from build123d import *

# Parameters (mm, degrees)
SKETCH1_W                                  = 120
SKETCH1_H                                  = 60
BOSS_EXTRUDE1_DEPTH                        = 10
CUT_EXTRUDE1_DEPTH                         = 71
CUT_EXTRUDE1_DEPTH_BACK                    = 71
SKETCH2_W                                  = 100
SKETCH2_H                                  = 10
FILLET1_R                                  = 5
SKETCH4_R                                  = 1.7
CUT_EXTRUDE3_DEPTH                         = 115.455231423
CUT_EXTRUDE4_DEPTH                         = 3
MIRROR1_AT_THE_SECOND_PLANE_COPY_1_SKETC_R = 1.7
MIRROR1_AT_THE_SECOND_PLANE_COPY_1_DEPTH   = 115.455231423
MIRROR1_AT_THE_SECOND_PLANE_COPY_2_DEPTH   = 3
MIRROR2_COPY_1_SKETCH_R                    = 1.7
MIRROR2_COPY_1_DEPTH                       = 115.455231423
MIRROR2_COPY_2_DEPTH                       = 3
MIRROR2_COPY_3_SKETCH_R                    = 1.7
MIRROR2_COPY_3_DEPTH                       = 115.455231423
MIRROR2_COPY_4_DEPTH                       = 3
MIRROR2_COPY_5_SKETCH_R                    = 1.7
MIRROR2_COPY_5_DEPTH                       = 115.455231423
MIRROR2_COPY_6_DEPTH                       = 3
MIRROR2_COPY_7_SKETCH_R                    = 1.7
MIRROR2_COPY_7_DEPTH                       = 115.455231423
SKETCH6_R                                  = 10
CUT_EXTRUDE5_DEPTH                         = 71


with BuildPart() as part:
    # Sketch1 → Boss-Extrude1 (new, symmetric)
    with BuildSketch(Plane.XY):
        Rectangle(SKETCH1_W, SKETCH1_H)
    extrude(amount=BOSS_EXTRUDE1_DEPTH, both=True)

    # Sketch2 → Cut-Extrude1 (cut, two sides: drawn at the far end of the back side and taken through both)
    with BuildSketch(Plane.XY.offset(10).offset(-CUT_EXTRUDE1_DEPTH_BACK)):
        with Locations((0, -25)):
            Rectangle(SKETCH2_W, SKETCH2_H)
        with Locations((0, 25)):
            Rectangle(SKETCH2_W, SKETCH2_H)
    extrude(amount=CUT_EXTRUDE1_DEPTH + CUT_EXTRUDE1_DEPTH_BACK, mode=Mode.SUBTRACT)

    # Fillet1
    fillet1_edges = [part.edges().sort_by_distance(p)[0] for p in [
        (55, -30, -10),
        (-55, 30, -10),
        (-55, -30, 10),
        (-55, 30, 10),
        (55, -30, 10),
        (-55, -30, -10),
        (55, 30, -10),
        (55, 30, 10),
    ]]
    fillet(fillet1_edges, radius=FILLET1_R)

    # Sketch4 → Cut-Extrude3 (cut, symmetric)
    with BuildSketch(Plane.ZY.offset(-50)):
        with Locations((-5, 25)):
            Circle(SKETCH4_R)
    cut_extrude3 = extrude(amount=CUT_EXTRUDE3_DEPTH, both=True, mode=Mode.SUBTRACT)

    # Sketch5 → Cut-Extrude4 (cut)
    with BuildSketch(Plane.ZY.offset(-50)):
        Polygon((-7.886751346, 25), (-6.443375673, 22.5), (-3.556624327, 22.5), (-2.113248654, 25), (-3.556624327, 27.5), (-6.443375673, 27.5), align=None)
    cut_extrude4 = extrude(amount=-CUT_EXTRUDE4_DEPTH, mode=Mode.SUBTRACT)

    # Mirror1: Cut-Extrude3, Cut-Extrude4 across plane
    add(cut_extrude3.mirror(Plane(origin=(0, 0, 0), x_dir=(0, 0, 1), z_dir=(1, 0, 0))), mode=Mode.SUBTRACT)
    add(cut_extrude4.mirror(Plane(origin=(0, 0, 0), x_dir=(0, 0, 1), z_dir=(1, 0, 0))), mode=Mode.SUBTRACT)

    # Mirror1 at the second plane: Cut-Extrude3, Cut-Extrude4 across plane
    add(cut_extrude3.mirror(Plane.XY), mode=Mode.SUBTRACT)
    add(cut_extrude4.mirror(Plane.XY), mode=Mode.SUBTRACT)

    # Mirror1 at the second plane copy 1 sketc → Mirror1 at the second plane copy 1 (cut, symmetric)
    with BuildSketch(Plane(origin=(-50, 0, 0), x_dir=(0, 0, -1), z_dir=(1, 0, 0))):
        with Locations((-5, 25)):
            Circle(MIRROR1_AT_THE_SECOND_PLANE_COPY_1_SKETC_R)
    extrude(amount=MIRROR1_AT_THE_SECOND_PLANE_COPY_1_DEPTH, both=True, mode=Mode.SUBTRACT)

    # Mirror1 at the second plane copy 2 sketc → Mirror1 at the second plane copy 2 (cut)
    with BuildSketch(Plane(origin=(-50, 0, 0), x_dir=(0, 0, -1), z_dir=(1, 0, 0))):
        Polygon((-7.886751346, 25), (-6.443375673, 22.5), (-3.556624327, 22.5), (-2.113248654, 25), (-3.556624327, 27.5), (-6.443375673, 27.5), align=None)
    extrude(amount=-MIRROR1_AT_THE_SECOND_PLANE_COPY_2_DEPTH, mode=Mode.SUBTRACT)

    # Mirror2: Cut-Extrude4 across plane
    add(cut_extrude4.mirror(Plane.ZX), mode=Mode.SUBTRACT)

    # Mirror2 copy 1 sketch → Mirror2 copy 1 (cut, symmetric)
    with BuildSketch(Plane(origin=(-50, 0, 0), x_dir=(0, 0, 1), z_dir=(1, 0, 0))):
        with Locations((-5, 25)):
            Circle(MIRROR2_COPY_1_SKETCH_R)
    extrude(amount=MIRROR2_COPY_1_DEPTH, both=True, mode=Mode.SUBTRACT)

    # Mirror2 copy 2 sketch → Mirror2 copy 2 (cut)
    with BuildSketch(Plane(origin=(-50, 0, 0), x_dir=(0, 0, 1), z_dir=(1, 0, 0))):
        Polygon((-7.886751346, 25), (-6.443375673, 22.5), (-3.556624327, 22.5), (-2.113248654, 25), (-3.556624327, 27.5), (-6.443375673, 27.5), align=None)
    extrude(amount=-MIRROR2_COPY_2_DEPTH, mode=Mode.SUBTRACT)

    # Mirror2 copy 3 sketch → Mirror2 copy 3 (cut, symmetric)
    with BuildSketch(Plane(origin=(50, 0, 0), x_dir=(0, 0, -1), z_dir=(-1, 0, 0))):
        with Locations((-5, 25)):
            Circle(MIRROR2_COPY_3_SKETCH_R)
    extrude(amount=MIRROR2_COPY_3_DEPTH, both=True, mode=Mode.SUBTRACT)

    # Mirror2 copy 4 sketch → Mirror2 copy 4 (cut)
    with BuildSketch(Plane(origin=(50, 0, 0), x_dir=(0, 0, -1), z_dir=(-1, 0, 0))):
        Polygon((-7.886751346, 25), (-6.443375673, 22.5), (-3.556624327, 22.5), (-2.113248654, 25), (-3.556624327, 27.5), (-6.443375673, 27.5), align=None)
    extrude(amount=-MIRROR2_COPY_4_DEPTH, mode=Mode.SUBTRACT)

    # Mirror2 copy 5 sketch → Mirror2 copy 5 (cut, symmetric)
    with BuildSketch(Plane(origin=(-50, 0, 0), x_dir=(0, 0, -1), z_dir=(1, 0, 0))):
        with Locations((-5, -25)):
            Circle(MIRROR2_COPY_5_SKETCH_R)
    extrude(amount=MIRROR2_COPY_5_DEPTH, both=True, mode=Mode.SUBTRACT)

    # Mirror2 copy 6 sketch → Mirror2 copy 6 (cut)
    with BuildSketch(Plane(origin=(-50, 0, 0), x_dir=(0, 0, -1), z_dir=(1, 0, 0))):
        Polygon((-7.886751346, -25), (-6.443375673, -22.5), (-3.556624327, -22.5), (-2.113248654, -25), (-3.556624327, -27.5), (-6.443375673, -27.5), align=None)
    extrude(amount=-MIRROR2_COPY_6_DEPTH, mode=Mode.SUBTRACT)

    # Mirror2 copy 7 sketch → Mirror2 copy 7 (cut, symmetric)
    with BuildSketch(Plane.ZY.offset(-50)):
        with Locations((-5, -25)):
            Circle(MIRROR2_COPY_7_SKETCH_R)
    extrude(amount=MIRROR2_COPY_7_DEPTH, both=True, mode=Mode.SUBTRACT)

    # Sketch6 → Cut-Extrude5 (cut, through all)
    with BuildSketch(Plane.XY.offset(10)):
        Circle(SKETCH6_R)
    extrude(amount=-CUT_EXTRUDE5_DEPTH, mode=Mode.SUBTRACT)


solid = part.part
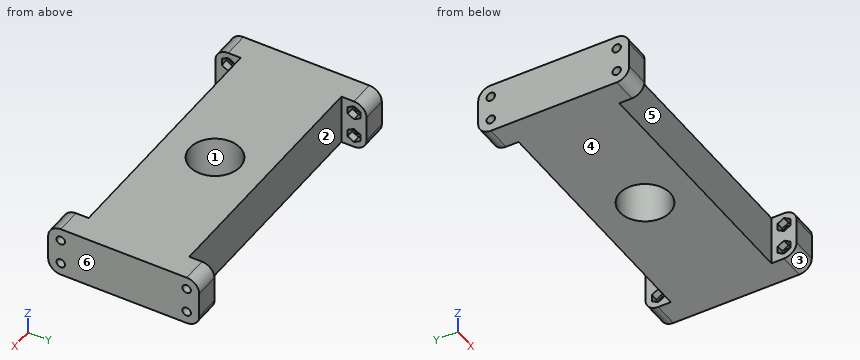
Verification items for the finished model (mm, model axes). Face numbers are marked on the shaded views. A direction names the side the tool comes from. Coordinates: 2 decimals unless noted, no trailing zeros. Loops run counter-clockwise (first coordinate to the right, second up) from the corner with the lowest first, then second, coordinate; pieces in that order, holes last. Notation, with made-up numbers: M 1.25,85 L 58.25,85 A29 cw 58.25,116 Z; hole C -4,-15 d9. An arc over 180 degrees is marked long. One line per item, written item: value.
1. Material ranges on line 1 along Y through (x, z) = (-54.5, -5); line 2 along X through (y, z) = (24, -2.5); line 3 along Y through (x, z) = (0, 1), recorded low to high. Write a range as from..to.
Answers follow:
line 1: -30..-26.7, -23.3..23.3, 26.7..30
line 2: -60..-50, 50..60
line 3: -20..-10, 10..20
2. Gauge pin test, flat ends, axial feed: P1, Ø1, axis at x = 35, z = 7, coming from the +Y side; P2, Ø1.5, axis at x = 11.5, z = -1, coming from the -Y side. Record the tip position at first contact, or that the pin passes through.
Answers follow:
P1: y = 20
P2: y = -20
3. Set-up check for the marked faces 5 and 6: record each of +Z, -Z, +X, -X, +Y, -Y from which the full face is reachable in a straight line by a thin tool's end or side.
Answers follow:
face 5: +Z, -Z, -Y
face 6: +Z, -Z, +X, +Y, -Y
4. Mould release check, pull along Y, two halves, no side actions. Record for the marked faces 1, 2, 3 and 4: pulls with the +Y half, pulls with the -Y half, needs draft (parallel to the pull), parting line crosses it, or undercut.
Answers follow:
face 1: undercut
face 2: pulls with the +Y half
face 3: pulls with the -Y half
face 4: needs draft
5. Section check A-A on y = 0. Record the cut outline in (x, z).
Answers follow:
outline: M -60,-10 L -10,-10 L -10,10 L -60,10 Z; M 10,-10 L 60,-10 L 60,10 L 10,10 Z
6. Section check C-C on x = 18.5. Record the cut outline in (y, z), plus the area to 3 significant figures.
Answers follow:
outline: M -20,-10 L 20,-10 L 20,10 L -20,10 Z
area: 800 mm^2
7. Section check B-B on x = 0. Record the cut outline in (y, z).
Answers follow:
outline: M -20,-10 L -10,-10 L -10,10 L -20,10 Z; M 10,-10 L 20,-10 L 20,10 L 10,10 Z
